from build123d import *

# Parameters (mm, degrees)
PAD_DEPTH      = 7
CYLINDER_R     = 1
CYLINDER_DEPTH = 10
ARRAY_X_COUNT  = 2
ARRAY_X_PITCH  = 66
ARRAY_Y_COUNT  = 2
ARRAY_Y_PITCH  = 16
BOX_W          = 56
BOX_H          = 26
BOX_DEPTH      = 5
BOX001_W       = 76
BOX001_H       = 28
BOX001_DEPTH   = 6
FILLET_R       = 5


with BuildPart() as wire_hole_body:
    # Sketch → Pad (new body)
    with BuildSketch(Plane.XZ):
        with BuildLine():
            Line((0, 5), (-10, 5))
            Line((-10, 5), (-10, 0.583155))
            add(Edge.make_bspline(
                [(-10, 0.583155), (-9.116008, 1.942432), (-7.251605, 3.386368), (-4.874426, 2.178075), (0, 0)],
                knots=[0, 0, 0, 0, 0.5, 1, 1, 1, 1], degree=3))
            Line((0, 0), (0, 5))
        make_face()
    extrude(amount=PAD_DEPTH)


with BuildPart() as part_mirroring:
    # Part__Mirroring: instance of wire hole body
    add(wire_hole_body.part.mirror(Plane(origin=(28, 0, 0), x_dir=(0, -1, 0), z_dir=(1, 0, 0))))


with BuildPart() as wire_hole_fusion:
    # Fusion001 base: copy of wire hole body
    add(wire_hole_body.part)

    # Fusion001: union Part__Mirroring
    add(part_mirroring.part)


with BuildPart() as wire_hole_fusion_1:
    # Fusion001 placement: moved
    add(wire_hole_fusion.part.moved(Location((0, 16.5, 0))))


with BuildPart() as screw_hole_array:
    # Cylinder → Cylinder (new body)
    with BuildSketch(Plane.XY):
        Circle(CYLINDER_R)
    extrude(amount=CYLINDER_DEPTH)

    # Array X: screw hole array ×2


with BuildPart() as screw_hole_array_1:
    add(screw_hole_array.part)
    with Locations(*[(i * ARRAY_X_PITCH, 0, 0) for i in range(1, ARRAY_X_COUNT)]):
        add(screw_hole_array.part)

    # Array Y: screw hole array ×2


with BuildPart() as screw_hole_array_2:
    add(screw_hole_array_1.part)
    with Locations(*[(0, i * ARRAY_Y_PITCH, 0) for i in range(1, ARRAY_Y_COUNT)]):
        add(screw_hole_array_1.part)


with BuildPart() as screw_hole_array_3:
    # Array placement: moved
    add(screw_hole_array_2.part.moved(Location((-5, 5, 0))))


with BuildPart() as extraction_fusion:
    # Box → Box (new body)
    with BuildSketch(Plane.XY):
        with Locations((28, 13)):
            Rectangle(BOX_W, BOX_H)
    extrude(amount=BOX_DEPTH)

    # Fusion: union wire hole fusion, screw hole array
    add(wire_hole_fusion_1.part)
    add(screw_hole_array_3.part)


with BuildPart() as box_cut:
    # Box001 → Box001 (new body)
    with BuildSketch(Plane(origin=(-10, -1, -1), x_dir=(1, 0, 0), z_dir=(0, 0, 1))):
        with Locations((38, 14)):
            Rectangle(BOX001_W, BOX001_H)
    extrude(amount=BOX001_DEPTH)

    # Fillet
    fillet_edges = [box_cut.edges().sort_by_distance(p)[0] for p in [
        (-10, -1, 2),
        (-10, 27, 2),
        (66, -1, 2),
        (66, 27, 2),
    ]]
    fillet(fillet_edges, radius=FILLET_R)

    # Cut: cut extraction fusion
    add(extraction_fusion.part, mode=Mode.SUBTRACT)


solid = box_cut.part
For this review, take the finished solid that the model builds, in its own axes (mm). A direction names the side the tool comes from. Give positions to 0.01 mm unless a question says otherwise; leave off trailing zeros. Order: outer loops, then holes, each group sorted by start corner. A loop starts at its lowest first (then second) coordinate and runs counter-clockwise, first axis right, second up. Notation, with made-up numbers: (-15, 76.25) -> (27, 76.25) arc R10 ccw to (27, 81.25) -> close; hole circle Ø10 at (-14.75, 14). An arc over 180 degrees is marked (long way). Write item = value, one per line.
1) Draft analysis for pull direction Y (two halves, no side actions). For faces 1 (the face through (-5, 6, 2)), 2 (the face through (25, -0.8, 5)), 3 (the face through (65, 25, 2)), state which applies: pulls with the +Y half, pulls with the -Y half, needs draft (parallel to the pull), parting line crosses it, or undercut.
Findings:
face_1 = undercut
face_2 = needs draft
face_3 = pulls with the +Y half
2) We need section C-C, the plane x = 32.5. Give the boundary of the cut face in (y, z), and give its area (3 significant figures).
Findings:
outline = (-1, -1) -> (27, -1) -> (27, 5) -> (26, 5) -> (26, 0) -> (0, 0) -> (0, 5) -> (-1, 5) -> close
area = 38.0 mm^2
3) To check wall thickness, follow L1, parallel to Y at x = -5, z = 1.1; L2, parallel to Y at x = -5, z = 3.2; L3, parallel to X at y = 21, z = 1.25. State the ranges of each line that lie inside material, in increasing order. Write a range as from..to.
Findings:
L1 = -1..4, 6..20, 22..27
L2 = -1..4, 6..9.5, 16.5..20, 22..27
L3 = -10..-6, -4..0, 56..60, 62..66
4) For faces 4 (the face through (-9, 1, 2)), 5 (the face through (-5, 9.5, 3)), list the 3-axis set-ups (+Z, -Z, +X, -X, +Y, -Y) from which the entire face can be reached by the end or side of a thin tool; tool diameter is ignored.
Findings:
face_4 = +Z, -Z, -X, -Y
face_5 = +Z
5) Insertion check: pin 1 (0.6 mm diameter, centred on x = -5, y = 21, fed in from +Z); pin 2 (2.5 mm diameter, centred on x = -5, y = 5, fed in from +Z); pin 3 (3 mm diameter, centred on x = 57, y = 14.5, fed in from +Z). Each pin has a flat end and moves straight along its axis. Give the tip position at first contact, or say it passes through.
Findings:
pin_1 = 0
pin_2 = 5
pin_3 = 1.12
6) We need section B-B, the plane y = 21. Give the boundary of the cut face in (x, z), and give its area (3 significant figures).
Findings:
outline = (-10, -1) -> (66, -1) -> (66, 5) -> (62, 5) -> (62, 0) -> (60, 0) -> (60, 5) -> (56, 5) -> (56, 0) -> (0, 0) -> (0, 5) -> (-4, 5) -> (-4, 0) -> (-6, 0) -> (-6, 5) -> (-10, 5) -> close
area = 156 mm^2
7) We need section A-A, the plane z = 4. Give the boundary of the cut face in (x, y), and give its area (3 significant figures).
Findings:
outline = (-10, 4) arc R5 ccw to (-5, -1) -> (61, -1) arc R5 ccw to (66, 4) -> (66, 9.5) -> (56, 9.5) -> (56, 0) -> (0, 0) -> (0, 9.5) -> (-10, 9.5) -> close; (-10, 16.5) -> (0, 16.5) -> (0, 26) -> (56, 26) -> (56, 16.5) -> (66, 16.5) -> (66, 22) arc R5 ccw to (61, 27) -> (-5, 27) arc R5 ccw to (-10, 22) -> close; hole circle Ø2 at (-5, 5); hole circle Ø2 at (-5, 21); hole circle Ø2 at (61, 5); hole circle Ø2 at (61, 21)
area = 498 mm^2
